Model file for the job. Use its own axes, mm. A direction names the side the tool comes from. Round coordinates to 2 decimals unless told otherwise and drop trailing zeros. Order: outer loops, then holes, each group sorted by start corner. A loop starts at its lowest first (then second) coordinate and runs counter-clockwise, first axis right, second up. Notation, with made-up numbers: (-40, 31.5) - (12, 31.5) arc R15 ccw to (12, 51.5) - close; hole circle Ø7 at (53, 33). An arc over 180 degrees is marked (long way). Put each result on its own line as item: value. Start each with the question number.
Item 1: Saw through at D-D on z = 5.25. List the corners of the cut face in (x, y), plus the area to 3 significant figures.
Item 2: Mould opens along X. For faces 6 (the face through (25.382, -18, 11)), 7 (the face through (-18, -10.135, 12)), 8 (the face through (21.907, -28.427, 12.727)) say: pulls with the +X half, pulls with the -X half, needs draft (parallel to the pull), parting line crosses it, or undercut.
Item 3: Pin check, flat tips, straight feed: pin 1 Ø4 at (x, z) = (-5, 13) entering from +Y; pin 2 Ø1 at (x, y) = (12, -23) entering from -Z; pin 3 Ø4 at (x, y) = (15.53, -7.92) entering from +Z. Stop position of each tip, or through.
Item 4: Saw through at A-A on z = 2.25. List the corners of the cut face in (x, y), plus the area to 3 significant figures.
Item 5: Saw through at B-B on x = -5.5. List the corners of the cut face in (y, z), plus the area to 3 significant figures.
Item 6: Which spindle directions (+Z, -Z, +X, -X, +Y, -Y) get a long thin tool onto all of the face, cutting with end or side? Do faces 1 (the face through (-10.868, -27, 2)), 2 (the face through (15, -25.811, 12)), 3 (the face through (-1, -30.074, 5)), 4 (the face through (12.529, -9, 12)), 5 (the face through (16.91, -7.48, 4.82)). Say none if no direction does.
Item 7: Probe probe 1 along Y at (x, z) = (-24, 6); probe 2 along X at (y, z) = (-8.25, 5.5); probe 3 along X at (y, z) = (-27, 2.25). List the from-to ranges inside material, lowest first.
Item 8: Saw through at C-C on y = -8.5. List the corners of the cut face in (x, z).
```python
from build123d import *

# Parameters (mm, degrees)
CROQUIS1_W                = 53
CROQUIS1_H                = 6.1
SALIENTE_EXTRUIR1_DEPTH   = 10
SALIENTE_EXTRUIR1_2_DEPTH = 10
CROQUIS2_W                = 53
CROQUIS2_H                = 24.2
SALIENTE_EXTRUIR2_DEPTH   = 5
CORTAR_EXTRUIR1_DEPTH     = 100
CROQUIS4_W                = 19.5
CROQUIS4_H                = 3.2
CORTAR_EXTRUIR2_DEPTH     = 10
CROQUIS5_W                = 6
CROQUIS5_H                = 4.263570071
CROQUIS5_H_2              = 4.260183182
CORTAR_EXTRUIR3_DEPTH     = 5.5
CROQUIS6_R                = 1.45
CORTAR_EXTRUIR4_DEPTH     = 20


with BuildPart() as part:
    # Croquis1 → Saliente-Extruir1 (new body)
    with BuildSketch(Plane.XY):
        with Locations((-1.118469745, -8.924349429)):
            Rectangle(CROQUIS1_W, CROQUIS1_H)
    extrude(amount=SALIENTE_EXTRUIR1_DEPTH)



with BuildPart() as body_2:
    # Croquis1 → Saliente-Extruir1 2 (new body)
    with BuildSketch(Plane.XY):
        with Locations((-1.118469745, -27.024349429)):
            Rectangle(CROQUIS1_W, CROQUIS1_H)
    extrude(amount=SALIENTE_EXTRUIR1_2_DEPTH)


with BuildPart() as part_1:
    add(part.part)

    add(body_2.part)  # Saliente-Extruir2 merges body 2
    # Croquis2 → Saliente-Extruir2 (add)
    with BuildSketch(Plane.XY.offset(10)):
        with Locations((-1.118469745, -17.974349429)):
            Rectangle(CROQUIS2_W, CROQUIS2_H)
    extrude(amount=SALIENTE_EXTRUIR2_DEPTH)

    # Croquis3 → Cortar-Extruir1 (cut)
    with BuildSketch(Plane.ZY.offset(27.618469745)):
        Polygon((10.51738062, -5.874349429), (15, -9.216602222), (15, -5.874349429), align=None)
        Polygon((15, -26.732096635), (15, -30.074349429), (10.51738062, -30.074349429), align=None)
    extrude(amount=-CORTAR_EXTRUIR1_DEPTH, mode=Mode.SUBTRACT)

    # Croquis4 → Cortar-Extruir2 (cut)
    with BuildSketch(Plane.XZ.offset(30.074349429)):
        with Locations((-1.118469745, 1.6)):
            Rectangle(CROQUIS4_W, CROQUIS4_H)
    extrude(amount=-CORTAR_EXTRUIR2_DEPTH, mode=Mode.SUBTRACT)

    # Croquis5 → Cortar-Extruir3 (cut)
    with BuildSketch(Plane.XY.offset(15)):
        with Locations((-17.765649999, -27.942564393)):
            Rectangle(CROQUIS5_W, CROQUIS5_H)
        with Locations((-17.765649999, -8.00444102)):
            Rectangle(CROQUIS5_W, CROQUIS5_H_2)
        with Locations((15.528710509, -27.942564393)):
            Rectangle(CROQUIS5_W, CROQUIS5_H)
        with Locations((15.528710509, -8.00444102)):
            Rectangle(CROQUIS5_W, CROQUIS5_H_2)
    extrude(amount=-CORTAR_EXTRUIR3_DEPTH, mode=Mode.SUBTRACT)

    # Croquis6 → Cortar-Extruir4 (cut)
    with BuildSketch(Plane.XY.offset(9.5)):
        with Locations((-17.765649999, -7.915512161)):
            Circle(CROQUIS6_R)
        with Locations((15.528710509, -7.915512161)):
            Circle(CROQUIS6_R)
        with Locations((15.528710509, -28.033186696)):
            Circle(CROQUIS6_R)
        with Locations((-17.765649999, -28.033186696)):
            Circle(CROQUIS6_R)
    extrude(amount=-CORTAR_EXTRUIR4_DEPTH, mode=Mode.SUBTRACT)


solid = part_1.part
```
Results found:
1. outline: (-27.62, -30.07) - (25.38, -30.07) - (25.38, -23.97) - (-27.62, -23.97) - close; (-27.62, -11.97) - (25.38, -11.97) - (25.38, -5.87) - (-27.62, -5.87) - close; hole circle Ø2.9 at (-17.77, -28.03); hole circle Ø2.9 at (-17.77, -7.92); hole circle Ø2.9 at (15.53, -28.03); hole circle Ø2.9 at (15.53, -7.92)
1. area: 620 mm²
2. face 6: pulls with the +X half
2. face 7: undercut
2. face 8: needs draft
3. pin 1: stops at y = -6.23
3. pin 2: stops at z = 10
3. pin 3: stops at z = 9.5
4. outline: (-27.62, -30.07) - (-10.87, -30.07) - (-10.87, -23.97) - (-27.62, -23.97) - close; (-27.62, -11.97) - (25.38, -11.97) - (25.38, -5.87) - (-27.62, -5.87) - close; (8.63, -30.07) - (25.38, -30.07) - (25.38, -23.97) - (8.63, -23.97) - close; hole circle Ø2.9 at (-17.77, -28.03); hole circle Ø2.9 at (-17.77, -7.92); hole circle Ø2.9 at (15.53, -28.03); hole circle Ø2.9 at (15.53, -7.92)
4. area: 501 mm²
5. outline: (-30.07, 3.2) - (-23.97, 3.2) - (-23.97, 10) - (-11.97, 10) - (-11.97, 0) - (-5.87, 0) - (-5.87, 10.52) - (-9.22, 15) - (-26.73, 15) - (-30.07, 10.52) - close
5. area: 208 mm²
6. face 1: -Z, -Y
6. face 2: +Z, -Y
6. face 3: +Z, -Z, +X, -X, -Y
6. face 4: +Z, +Y
6. face 5: +Z, -Z
7. probe 1: y = -30.07 to -23.97, -11.97 to -5.87
7. probe 2: x = -27.62 to -19.18, -16.35 to 14.12, 16.94 to 25.38
7. probe 3: x = -27.62 to -18.78, -16.75 to -10.87, 8.63 to 14.51, 16.55 to 25.38
8. outline: (-27.62, 0) - (-19.09, 0) - (-19.09, 9.5) - (-20.77, 9.5) - (-20.77, 14.04) - (-27.62, 14.04) - close; (-16.44, 0) - (14.2, 0) - (14.2, 9.5) - (12.53, 9.5) - (12.53, 14.04) - (-14.77, 14.04) - (-14.77, 9.5) - (-16.44, 9.5) - close; (16.86, 0) - (25.38, 0) - (25.38, 14.04) - (18.53, 14.04) - (18.53, 9.5) - (16.86, 9.5) - close
